Check sheet for the modelled part. Datum: model origin and axes. Units: mm. A direction names the side the tool comes from. Round coordinates to 2 decimals unless told otherwise and drop trailing zeros. Write each loop counter-clockwise with the first axis right and the second up, starting at its lowest first coordinate (ties: lowest second). Pieces come first, ordered by that corner, then holes.
Item 1: Cross-section at C-C on z = -1081. Enter the section's corners in (x, y).
Item 2: Tool access check on faces 1 (the flat face through (1.588, 38, -601)), 2 (the flat face through (0, 38, -601)), 3 (the flat face through (7, 76.2, -618)). Record the directions out of +Z, -Z, +X, -X, +Y, -Y that give a thin tool (end or side, any length) a straight path to the whole face; none if there is none.
Item 3: Release check for a two-part mould opening along Y. For faces 4 (the flat face through (-7, 38, 0)), 5 (the flat face through (7, 0, -601)), 6 (the cylindrical face through (0.8, 47.76, -293.86)) record: +Y half, -Y half, draft (parallel to the pull), parting line (faces both ways), or undercut.
Item 4: Go/stop test with flat-tipped pins: pin 1 Ø23 at (y, z) = (44, -909) entering from -X; pin 2 Ø23 at (y, z) = (38.1, -913.21) entering from -X; pin 3 Ø5.5 at (x, y) = (-4, 37) entering from +Z. Record where each tip stops, or that it passes through.
Item 5: Cross-section at A-A on y = 38.1. Enter the section's corners in (x, z).
Item 6: Cross-section at B-B on x = 10.25. Enter the section's corners in (y, z).
Item 7: Material ranges on line 1 (Z direction, x = 1.05, y = 38.1); line 2 (Z direction, x = -7.25, y = 57.5); line 3 (Y direction, x = 2.5, z = -757), recorded low to high.
Autodesk Inventor part; units mm, degrees
ref_plane "YZ Plane" through (0, 0, 0) normal (1, 0, 0) x (0, 1, 0)
ref_plane "XZ Plane" through (0, 0, 0) normal (0, 1, 0) x (-1, 0, 0)
ref_plane "XY Plane" through (0, 0, 0) normal (0, 0, 1) x (1, 0, 0)
sketch "Sketch1" plane through (0, 0, 0) normal (1, 0, 0) x (0, 1, 0)
  line L0 (0, 0) -> (76.2, 0)
  line L1 (76.2, 0) -> (76.2, -1219.2)
  line L2 (76.2, -1219.2) -> (0, -1219.2)
  line L3 (0, -1219.2) -> (0, 0)
  dimension "d0" = 76.2
  dimension "d1" = 1219.2
extrude "Extrusion1" add sketch "Sketch1" along normal blind 1.5875
sketch "Sketch2" plane through (0, 0, 0) normal (0, 0, 1) x (1, 0, 0)
  line L0 (0, 76.2) -> (0, 0)
  line L1 (0, 0) -> (1.5875, 0)
  line L2 (1.5875, 76.2) -> (1.5875, 0)
  line L3 (0, 76.2) -> (1.5875, 76.2)
  line L4 (1.5875, 0) -> (-11.1125, 0)
  line L5 (-11.1125, 0) -> (-11.1125, 76.2)
  line L6 (-11.1125, 76.2) -> (1.5875, 76.2)
  line L7 (1.5875, 76.2) -> (1.5875, 0)
  dimension "d4" = 12.7
extrude "Extrusion2" add sketch "Sketch2" against normal blind 1.5875 contours L0 L4 L5 L6
sketch "Sketch3" plane through (0, 0, -1219.2) normal (0, 0, -1) x (-1, 0, 0)
  line L0 (0, 0) -> (11.1125, 0)
  line L1 (11.1125, 0) -> (11.1125, 76.2)
  line L2 (11.1125, 76.2) -> (0, 76.2)
  line L3 (0, 0) -> (0, 76.2)
extrude "Extrusion3" add sketch "Sketch3" against normal blind 1.5875
sketch "Sketch5" plane through (1.5875, 76.2, 0) normal (0, 1, 0) x (1, 0, 0)
  line L0 (-1.5875, 1217.6125) -> (-1.5875, 1.5875)
  line L1 (-12.7, 1.5875) -> (-1.5875, 1.5875)
  line L2 (-12.7, 0) -> (-12.7, 1.5875)
  line L3 (-12.7, 0) -> (0, 0)
  line L4 (0, 1219.2) -> (0, 0)
  line L5 (-12.7, 1219.2) -> (0, 1219.2)
  line L6 (-12.7, 1219.2) -> (-12.7, 1217.6125)
  line L7 (-1.5875, 1217.6125) -> (-12.7, 1217.6125)
  line L8 (0, 0) -> (12.7, 0)
  line L9 (12.7, 0) -> (12.7, 1219.2)
  line L10 (12.7, 1219.2) -> (0, 1219.2)
  line L11 (0, 1219.2) -> (0, 0)
  point P0 (-1.5875, 0)
  dimension "d13" = 12.7
extrude "Extrusion4" add sketch "Sketch5" against normal blind 1.5875 contours L10 L9 L8 L4
sketch "Sketch6" plane through (1.5875, 0, -1219.2) normal (0, -1, 0) x (1, 0, 0)
  line L0 (12.7, 0) -> (12.7, 1219.2)
  line L1 (12.7, 1219.2) -> (0, 1219.2)
  line L2 (0, 0) -> (0, 1219.2)
  line L3 (0, 0) -> (12.7, 0)
  point P0 (-1.5875, 1219.2)
extrude "Extrusion5" add sketch "Sketch6" against normal blind 1.5875
sketch "Sketch7" plane through (1.5875, 0, 0) normal (1, 0, 0) x (0, 0, -1)
  line L0 (0, 1.5875) -> (1219.2, 1.5875)
  line L1 (1219.2, 1.5875) -> (1219.2, 74.6125)
  line L2 (1219.2, 74.6125) -> (0, 74.6125)
  line L3 (0, 74.6125) -> (0, 1.5875)
  line L4 (0, 38.1) -> (1217.6125, 38.1)
  line L5 (1217.6125, 76.2) -> (1217.6125, 0)
  line L6 (608.8062, 38.1) -> (608.8062, 66.0202)
  line L7 (608.8062, 66.0202) -> (0, 66.0202)
  line L8 (304.4031, 66.0202) -> (304.4031, 38.1)
  circle A0 centre (304.4031, 38.1) radius 14.3002
  circle A1 centre (608.8062, 38.1) radius 14.3002
  circle A2 centre (913.2094, 38.1) radius 14.3002
  point P0 (0, 0)
  dimension "d18" = 28.6004
  dimension "d19" = 28.6004
extrude "Extrusion6" cut sketch "Sketch7" against normal blind 25.4 contours A0 L8 L4 | L4 A0 | A2 L4 | L4 A2 | L8 A0 L4
properties part number "Chassis SideV1"
Response values:
1. outline: (0, 0) - (14.29, 0) - (14.29, 1.59) - (1.59, 1.59) - (1.59, 74.61) - (14.29, 74.61) - (14.29, 76.2) - (0, 76.2) - close
2. face 1: +Z, -Z, +X
2. face 2: -X, +Y, -Y
2. face 3: +Z, -Z, +X, -X, +Y
3. face 4: draft
3. face 5: -Y half
3. face 6: undercut
4. pin 1: stops at x = 0
4. pin 2: passes through
4. pin 3: stops at z = 0
5. outline: (-11.11, -1219.2) - (1.59, -1219.2) - (1.59, -927.51) - (0, -927.51) - (0, -1217.61) - (-11.11, -1217.61) - close; (-11.11, -1.59) - (0, -1.59) - (0, -290.1) - (1.59, -290.1) - (1.59, 0) - (-11.11, 0) - close; (0, -898.91) - (1.59, -898.91) - (1.59, -318.7) - (0, -318.7) - close
6. outline: (0, -1219.2) - (1.59, -1219.2) - (1.59, 0) - (0, 0) - close; (74.61, -1219.2) - (76.2, -1219.2) - (76.2, 0) - (74.61, 0) - close
7. line 1: z = -1219.2 to -927.51, -898.91 to -318.7, -290.1 to 0
7. line 2: z = -1219.2 to -1217.61, -1.59 to 0
7. line 3: y = 0 to 1.59, 74.61 to 76.2
